Input: part model. Units: mm. Frame: model coordinates. Face numbers are marked on the shaded views. A direction names the side the tool comes from. Give positions to 0.01 mm unless a question says otherwise; leave off trailing zeros. Loops run counter-clockwise (first coordinate to the right, second up) from the corner with the lowest first, then second, coordinate; pieces in that order, holes last. Notation, with made-up numbers: (68, 38.25) -> (80, 38.25) arc R27 ccw to (80, 57.25) -> close; hole circle Ø6 at (89.25, 56). An arc over 180 degrees is marked (long way). Use CSV: the item, a comma, the result in double quotes.
```python
from build123d import *

# Parameters (mm, degrees)
F0_R     = 3.5
F2_R     = 2.895
F4_R     = 4.25
F5_DEPTH = 1
F6_R     = 4.865
F7_DEPTH = 0.5


with BuildPart() as f3:
    # F0 (on Top) → F3 section 0
    with BuildSketch(Plane.XY):
        Circle(F0_R)
    # F2 (on offset) → F3 section 1
    with BuildSketch(Plane.XY.offset(9.5)):
        Circle(F2_R)
    loft()

    # F4 (on face) → F5 (join)
    with BuildSketch(Plane(origin=(0, 0, 0), x_dir=(1, 0, 0), z_dir=(0, 0, -1))):
        Circle(F4_R)
    extrude(amount=F5_DEPTH)

    # F6 (on face) → F7 (join)
    with BuildSketch(Plane(origin=(0, 0, -1), x_dir=(1, 0, 0), z_dir=(0, 0, -1))):
        Circle(F6_R)
    extrude(amount=F7_DEPTH)


solid = f3.part
```
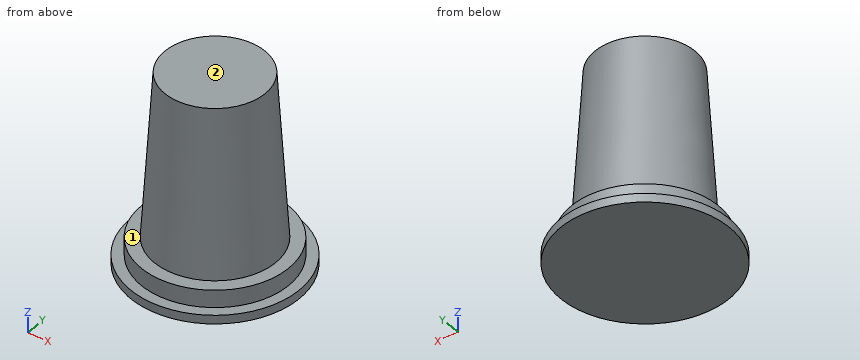
1) Section query A-A (x = 0). Return loops of the section in (y, z) (3 decimals).
From the geometry:
outline,"(-4.865, -1.5) -> (4.865, -1.5) -> (4.865, -1) -> (4.25, -1) -> (4.25, 0) -> (3.5, 0) -> (2.895, 9.5) -> (-2.895, 9.5) -> (-3.5, 0) -> (-4.25, 0) -> (-4.25, -1) -> (-4.865, -1) -> close"
2) Section query D-D (z = 3.5). Return loops of the section in (x, y), then the cut area to 3 significant figures.
From the geometry:
outline,"circle Ø6.55 at (0, 0)"
area,"33.7 mm^2"
3) Section query B-B (y = 4). Return loops of the section in (x, z), then the cut area to 3 significant figures.
From the geometry:
outline,"(-2.77, -1.5) -> (2.77, -1.5) -> (2.77, -1) -> (1.44, -1) -> (1.44, 0) -> (-1.44, 0) -> (-1.44, -1) -> (-2.77, -1) -> close"
area,"5.64 mm^2"
4) Ray query, line 1 (Z direction, x = -3.75, y = 0.5); line 2 (Y direction, x = 0, z = -0.5); line 3 (X direction, y = -2.75, z = 4.25). Return the intervals inside material, ascending.
From the geometry:
line 1,"z = -1.5 to 0"
line 2,"y = -4.25 to 4.25"
line 3,"x = -1.69 to 1.69"
5) Contact query for flat-ended pins moving along their axis: pin 1 (1 mm diameter, centred on x = -1.5, y = -3, fed in from +Z); pin 2 (4 mm diameter, centred on y = -3.5, z = 3, fed in from -X); pin 3 (1.5 mm diameter, centred on x = -2, z = 2, fed in from -Y); pin 4 (3 mm diameter, centred on x = -0.5, z = 7.5, fed in from +Y). Output: stop coordinate, or through.
From the geometry:
pin 1,"stops at z = 9.5"
pin 2,"stops at x = -2.96"
pin 3,"stops at y = -3.14"
pin 4,"stops at y = 3.11"
6) Section query C-C (z = -0.5). Return loops of the section in (x, y).
From the geometry:
outline,"circle Ø8.5 at (0, 0)"
7) Reachability of the marked faces 1 and 2 from +Z, -Z, +X, -X, +Y, -Y: full face, straight path, thin tool, end or side. Return the list, or none.
From the geometry:
face 1,"+Z"
face 2,"+Z, +X, -X, +Y, -Y"
